```python
from build123d import *

# Parameters (mm, degrees)
EXTRUDE_1_DEPTH      = 3
SKETCH_9_R           = 3.5
SKETCH_9_R_2         = 1.65
CUT_EXTRUDE_5_DEPTH  = 6
CUT_EXTRUDE_START    = -1
CUT_EXTRUDE_7_DEPTH  = 87.53280603
SKETCH_13_R          = 0.55
CUT_EXTRUDE_10_DEPTH = 88.53280603


with BuildPart() as part:
    # Sketch 1 → Extrude 1 (new body)
    with BuildSketch(Plane.XY):
        with BuildLine():
            Line((0.000249999, 5.999750001), (14.999750012, 5.999750001))
            ThreePointArc((14.999750012, 5.999750001), (18.061380786, 6.60878139), (20.656854249, 8.343145751))
            Line((20.656854249, 8.343145751), (63.083261121, 50.769552622))
            ThreePointArc((63.083261121, 50.769552622), (69.093668761, 50.769552622), (69.093668761, 44.759144982))
            Line((69.093668761, 44.759144982), (20.647045788, -3.658779955))
            ThreePointArc((20.647045788, -3.658779955), (18.052240297, -5.391739688), (14.991867742, -6.000249999))
            Line((14.991867742, -6.000249999), (0.000249999, -6.000249999))
            ThreePointArc((0.000249999, -6.000249999), (-5.999750001, -0.000249999), (0.000249999, 5.999750001))
        make_face()
    extrude(amount=EXTRUDE_1_DEPTH)

    # Sketch 9 → Cut-Extrude 5 (cut)
    with BuildSketch(Plane.XY.offset(3)):
        Circle(SKETCH_9_R)
        with Locations((66.088464941, 47.764348802)):
            Circle(SKETCH_9_R_2)
    extrude(amount=-CUT_EXTRUDE_5_DEPTH, mode=Mode.SUBTRACT)

    # Sketch 9_4 → Cut-Extrude 7 (cut, through all)
    with BuildSketch(Plane.XY.offset(3).offset(CUT_EXTRUDE_START)):
        with BuildLine():
            Line((14.2, 1.55872543), (2.168203804, 2.747524752))
            ThreePointArc((2.168203804, 2.747524752), (3.149501017, 1.526644472), (3.5, 0))
            ThreePointArc((3.5, 0), (3.149501017, -1.526644472), (2.168203804, -2.747524752))
            Line((2.168203804, -2.747524752), (14.2, -1.94127457))
            ThreePointArc((14.2, -1.94127457), (15.785612929, -0.19127457), (14.2, 1.55872543))
        make_face()
    extrude(amount=-CUT_EXTRUDE_7_DEPTH, mode=Mode.SUBTRACT)

    # Sketch 13 → Cut-Extrude 10 (cut, through all)
    with BuildSketch(Plane.XY.offset(3)):
        with Locations((4.085, 0)):
            Circle(SKETCH_13_R)
        with Locations((6.085, 0)):
            Circle(SKETCH_13_R)
        with Locations((8.085, 0)):
            Circle(SKETCH_13_R)
        with Locations((10.085, 0)):
            Circle(SKETCH_13_R)
    extrude(amount=-CUT_EXTRUDE_10_DEPTH, mode=Mode.SUBTRACT)


solid = part.part
```
Part model, mm, in its own coordinate system. A direction names the side the tool comes from. Round coordinates to 2 decimals unless told otherwise and drop trailing zeros. Order: outer loops, then holes, each group sorted by start corner. A loop starts at its lowest first (then second) coordinate and runs counter-clockwise, first axis right, second up. Notation, with made-up numbers: M -11,-31.5 L 24,-31.5 A19 cw 24,-9.5 Z; hole C 4,35.25 d9. An arc over 180 degrees is marked long. Answer in a Markdown table with one row per item. Add a question column.
Q1. Mould opens along Y. For faces 1 (the face through (8.1, -2.35, 1.01)), 2 (the face through (7, 6, 1)), 3 (the face through (32, 19, 3)) say: +Y half, -Y half, draft (parallel to the pull), parting line (faces both ways), or undercut.
Q2. Cut at C-C on y = 22. Give the cut face in (x, z).
Q3. Pin check, flat tips, straight feed: pin 1 (1.8 mm diameter, centred on x = 4.085, y = 0, fed in from -Z); pin 2 (1.5 mm diameter, centred on x = 40.5, z = 2.5, fed in from +Y). Stop position of each tip, or through.
Q4. Cut at B-B on x = 36. Give the cut face in (y, z), and give its area (3 significant figures).
Q5. Wall check: L1, parallel to Y at x = 0, z = 0.75; L2, parallel to Y at x = 14, z = 0.4; L3, parallel to X at y = 2, z = 2.1. Give the ranges that are in metal, low to high. Write a range as from..to.
Q6. Cut at A-A on z = 1.15. Give the cut face in (x, y).
Q7. 3-axis set-ups, long thin cutter, end or side, ignore diameter. For faces 4 (the face through (8.268, 2.145, 1.014)), 5 (the face through (-6, 0, 1)): which of +Z, -Z, +X, -X, +Y, -Y reach the whole face in a straight line?
Established:
| question | item | result |
|---|---|---|
| 1 | face 1 | undercut |
| 1 | face 2 | +Y half |
| 1 | face 3 | draft |
| 2 | outline | M 34.31,0 L 46.32,0 L 46.32,3 L 34.31,3 Z |
| 3 | pin 1 | stops at z = 2 |
| 3 | pin 2 | stops at y = 28.94 |
| 4 | outline | M 11.69,0 L 23.69,0 L 23.69,3 L 11.69,3 Z |
| 4 | area | 36.0 mm2 |
| 5 | L1 | y = -6..-3.5, 3.5..6 |
| 5 | L2 | y = -6..-1.95, 1.58..6 |
| 5 | L3 | x = -5.66..-2.87, 2.87..26.31 |
| 6 | outline | M 0,-6 L 14.99,-6 A8 ccw 20.65,-3.66 L 69.09,44.76 A4.25 ccw 63.08,50.77 L 20.66,8.34 A8 cw 15,6 L 0,6 A6 ccw Z; hole M 2.17,-2.75 L 14.2,-1.94 A1.76 ccw 14.2,1.56 L 2.17,2.75 A3.5 ccw long Z; hole C 66.09,47.76 d3.3 |
| 7 | face 4 | -Z |
| 7 | face 5 | +Z, -Z, -X |
